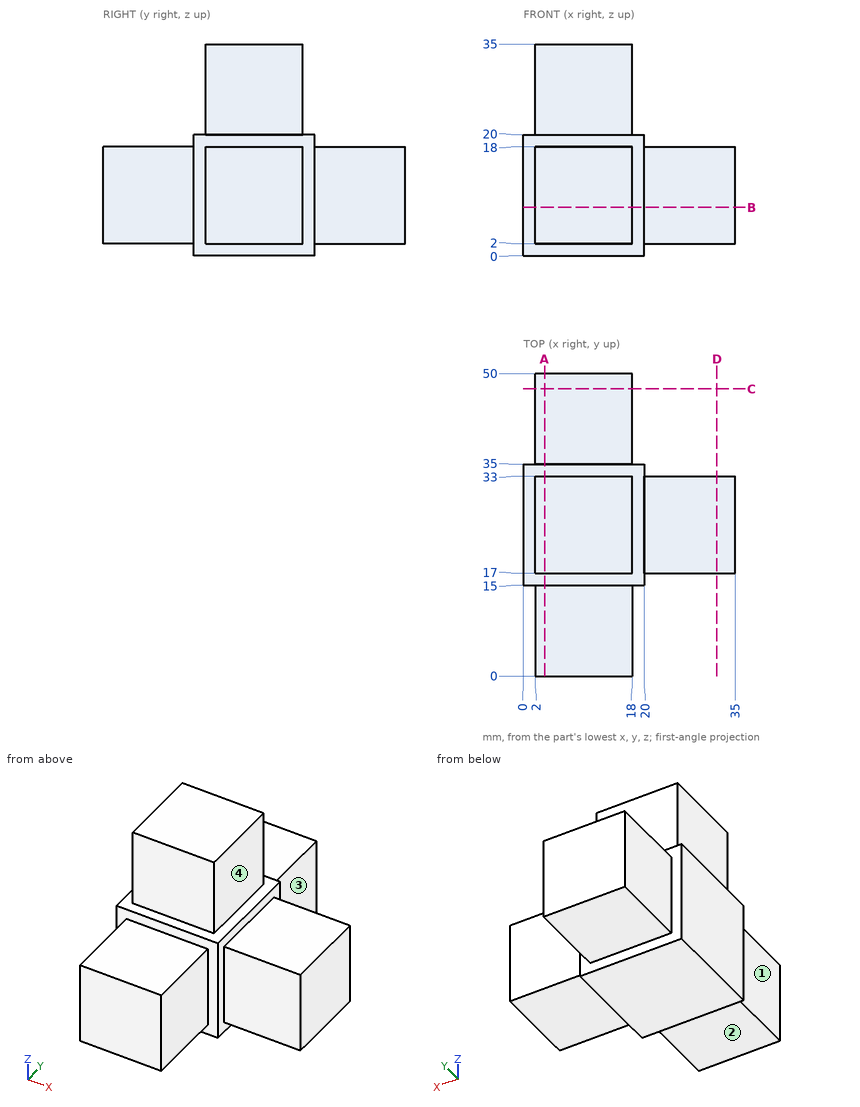
For this review, use the dimensioned drawing (mm, ordinates from the lowest corner) and the shaded views. A direction names the side the tool comes from. Give positions to 0.01 mm unless a question says otherwise; leave off trailing zeros. Loops run counter-clockwise (first coordinate to the right, second up) from the corner with the lowest first, then second, coordinate; pieces in that order, holes last.
Item 1: Tool access review of the marked faces 1, 2, 3 and 4: name each direction out of +Z, -Z, +X, -X, +Y, -Y from which nothing blocks a thin tool from reaching the whole face with its end or side.
Item 2: Take a section at B-B, the plane z = 8. State the section outline as (x, y) points.
Item 3: Take a section at A-A, the plane x = 3.5. State the section outline as (y, z) points.
Item 4: Take a section at C-C, the plane y = 47.5. State the section outline as (x, z) points, and give its area (3 significant figures).
Item 5: Insertion check: pin 1 (8 mm diameter, centred on x = 9.5, z = 27, fed in from +Y); pin 2 (7.5 mm diameter, centred on y = 40.5, z = 10.5, fed in from -X); pin 3 (3 mm diameter, centred on x = 5, y = 11, fed in from -Z). Each pin has a flat end and moves straight along its axis. Give the tip position at first contact, or say it passes through.
Item 6: For line 1 along X through (y, z) = (17.5, 23); line 2 along Y through (x, z) = (27.5, 7), list the stretches that pass through material, from the lowest coordinate up.
Item 7: Take a section at D-D, the plane x = 32. State the section outline as (y, z) points, and give its area (3 significant figures).
Calculated:
1. face 1: +Z, -Z, -X, -Y
1. face 2: -Z, +X, -X, -Y
1. face 3: +Z, -Z, +X, +Y
1. face 4: +Z, +X, +Y, -Y
2. outline: (0, 15) - (2, 15) - (2, 0) - (18, 0) - (18, 15) - (20, 15) - (20, 17) - (35, 17) - (35, 33) - (20, 33) - (20, 35) - (18, 35) - (18, 50) - (2, 50) - (2, 35) - (0, 35) - close
3. outline: (0, 2) - (15, 2) - (15, 0) - (35, 0) - (35, 2) - (50, 2) - (50, 18) - (35, 18) - (35, 20) - (33, 20) - (33, 35) - (17, 35) - (17, 20) - (15, 20) - (15, 18) - (0, 18) - close
4. outline: (2, 2) - (18, 2) - (18, 18) - (2, 18) - close
4. area: 256 mm2
5. pin 1: stops at y = 33
5. pin 2: stops at x = 2
5. pin 3: stops at z = 2
6. line 1: x = 2 to 18
6. line 2: y = 17 to 33
7. outline: (17, 2) - (33, 2) - (33, 18) - (17, 18) - close
7. area: 256 mm2
